Here's how the part is built. I have some questions about the finished solid (model axes, mm). A direction names the side the tool comes from. Coordinates: 2 decimals unless noted, no trailing zeros. Write each loop counter-clockwise with the first axis right and the second up, starting at its lowest first coordinate (ties: lowest second). Pieces come first, ordered by that corner, then holes. Notation, with made-up numbers: (28.5, -36) -> (68.5, -36) arc R33 ccw to (68.5, -1) -> close; hole circle Ø6 at (22, 35.5). An arc over 180 degrees is marked (long way). Use CSV: the item, a comma, the result in double quotes. Start each with the question number.
```python
from build123d import *

# Parameters (mm, degrees)
SKETCH_1_W                = 42
SKETCH_1_H                = 90
HOUSING_ENVELOPE_DEPTH    = 38
SKETCH_2_W                = 34
SKETCH_2_H                = 82
FRONT_ACCESS_WINDOW_DEPTH = 32
SKETCH_3_R                = 6.5
AXIAL_PASSAGE_DEPTH       = 107.339080304


with BuildPart() as part:
    # 草图1 → Housing_envelope (new body)
    with BuildSketch(Plane.XY):
        with Locations((21, 45)):
            Rectangle(SKETCH_1_W, SKETCH_1_H)
    extrude(amount=HOUSING_ENVELOPE_DEPTH)

    # 草图2 → Front_access_window (cut)
    with BuildSketch(Plane.XY.offset(38)):
        with Locations((21, 45)):
            Rectangle(SKETCH_2_W, SKETCH_2_H)
    extrude(amount=-FRONT_ACCESS_WINDOW_DEPTH, mode=Mode.SUBTRACT)

    # 草图3 → Axial_passage (cut, through all)
    with BuildSketch(Plane(origin=(0, 90, 0), x_dir=(1, 0, 0), z_dir=(0, 1, 0))):
        with Locations(Location((21, -19, 0), (0, 0, 270))):
            Circle(SKETCH_3_R)
    extrude(amount=-AXIAL_PASSAGE_DEPTH, mode=Mode.SUBTRACT)


solid = part.part
```
Item 1: I want a section at B-B on z = 19. Please give me the cut outline in (x, y).
Item 2: If I drill on line 1 along X through (y, z) = (55, 33.5); line 2 along X through (y, z) = (2.15, 19); line 3 along Y through (x, z) = (25.5, 27.5), over which ranges is the centre line in solid material (lowest first)?
Item 3: I want a section at C-C on x = 10.5. Please give me the cut outline in (y, z), then the cut area to 3 significant figures.
Item 4: I want a section at D-D on y = 73. Please give me the cut outline in (x, z), then the cut area to 3 significant figures.
Item 5: Thinking about a two-plate mould opening in Z: for faces 3 (the cylindrical face through (21.286, 2.028, 12.506)), 4 (the flat face through (16, 0, 14.5)), 5 (the flat face through (3.8, 48.5, 38)), which applies, +Z half, -Z half, draft (parallel to the pull), parting line (faces both ways), or undercut?
Item 6: I'm going to push a flat-ended pin straight in: pin 1 (17 mm diameter, centred on x = 20.5, y = 63, fed in from +Z). Where does the tip first touch, or does it pass through?
Item 7: I want a section at A-A on x = 21. Please give me the cut outline in (y, z).
Item 8: Which directions (+Z, -Z, +X, -X, +Y, -Y) give clear straight access to the entire face, cutting with the end or side of a thin tool? Please do faces 1 (the flat face through (21, 46, 0)), 2 (the flat face through (38, 44, 22)).
Geometry says:
1,outline,"(0, 0) -> (14.5, 0) -> (14.5, 4) -> (4, 4) -> (4, 86) -> (14.5, 86) -> (14.5, 90) -> (0, 90) -> close; (27.5, 0) -> (42, 0) -> (42, 90) -> (27.5, 90) -> (27.5, 86) -> (38, 86) -> (38, 4) -> (27.5, 4) -> close"
2,line 1,"0 to 4, 38 to 42"
2,line 2,"0 to 14.5, 27.5 to 42"
2,line 3,"0 to 4, 86 to 90"
3,outline,"(0, 0) -> (90, 0) -> (90, 38) -> (86, 38) -> (86, 6) -> (4, 6) -> (4, 38) -> (0, 38) -> close"
3,area,"796 mm2"
4,outline,"(0, 0) -> (42, 0) -> (42, 38) -> (38, 38) -> (38, 6) -> (4, 6) -> (4, 38) -> (0, 38) -> close"
4,area,"508 mm2"
5,face 3,"undercut"
5,face 4,"draft"
5,face 5,"+Z half"
6,pin 1,"z = 6"
7,outline,"(0, 0) -> (90, 0) -> (90, 12.5) -> (86, 12.5) -> (86, 6) -> (4, 6) -> (4, 12.5) -> (0, 12.5) -> close; (0, 25.5) -> (4, 25.5) -> (4, 38) -> (0, 38) -> close; (86, 25.5) -> (90, 25.5) -> (90, 38) -> (86, 38) -> close"
8,face 1,"-Z, +X, -X, +Y, -Y"
8,face 2,"+Z"
